Read the model definition and answer for the solid it produces. Units are mm, in the model's axes. A direction names the side the tool comes from. Round coordinates to 2 decimals unless told otherwise and drop trailing zeros. Write each loop counter-clockwise with the first axis right and the second up, starting at its lowest first coordinate (ties: lowest second). Pieces come first, ordered by that corner, then holes. Notation, with made-up numbers: (52.5, 23) - (104.5, 23) arc R22 cw to (104.5, 48) - close; hole circle Ø11 at (62, 43). An arc over 180 degrees is marked (long way). One line per item, written item: value. Start each with the question number.
(1) A cutting plane is placed at A-A, the plane x = -11. Determine the outline of the cut face in (y, z), plus the area to 3 significant figures.
(2) Find the intervals of material crossed by L1, parallel to Y at x = 12.5, z = 9.25; L2, parallel to Z at x = 31, y = -2.4; L3, parallel to X at y = -0.05, z = 0.5, in increasing order.
(3) A cutting plane is placed at C-C, the plane y = -2.3. Determine the outline of the cut face in (x, z).
(4) A cutting plane is placed at B-B, the plane z = 0. Determine the outline of the cut face in (x, y).
(5) For faces 1 (the face through (0, -2, 8)), 2 (the face through (-40.498, -1.986, 0.176)), 3 (the face through (40.498, -1.986, -0.176)), 4 (the face through (0, -2, -8)), determine the directions among +Z, -Z, +X, -X, +Y, -Y from which every point of the face is accessible in a straight line to the end or side of a thin tool.
(6) A flat-ended cylindrical pin translates along its axis: pin 1 Ø0.6 at (x, y) = (-7, -2.5) entering from -Z. Find the tip coordinate at first contact, or state that the pin passes through.
from build123d import *

# Parameters (mm, degrees)
F1_DEPTH = 1
F2_DEPTH = 3


with BuildPart() as f1:
    # F0 (on Front) → F1 (new body)
    with BuildSketch(Plane.XZ):
        with BuildLine():
            Line((-32.5, 8.5), (-32.5, 10.1))
            ThreePointArc((-32.5, 10.1), (-42.6, 0), (-32.5, -10.1))
            Line((-32.5, -10.1), (32.5, -10.1))
            Line((32.5, -10.1), (32.5, -8.5))
            Line((32.5, -8.5), (-32.5, -8.5))
            ThreePointArc((-32.5, -8.5), (-41, 0), (-32.5, 8.5))
        make_face()
        with BuildLine():
            Line((32.5, 10.1), (-32.5, 10.1))
            Line((-32.5, 10.1), (-32.5, 8.5))
            Line((-32.5, 8.5), (32.5, 8.5))
            ThreePointArc((32.5, 8.5), (41, 0), (32.5, -8.5))
            Line((32.5, -8.5), (32.5, -10.1))
            ThreePointArc((32.5, -10.1), (42.6, 0), (32.5, 10.1))
        make_face()
        with BuildLine():
            Line((32.5, 8.5), (-32.5, 8.5))
            Line((-32.5, 8.5), (-32.5, 8))
            Line((-32.5, 8), (32.5, 8))
            ThreePointArc((32.5, 8), (40.5, 0), (32.5, -8))
            Line((32.5, -8), (32.5, -8.5))
            ThreePointArc((32.5, -8.5), (41, 0), (32.5, 8.5))
        make_face()
        with BuildLine():
            Line((-32.5, 8), (-32.5, 8.5))
            ThreePointArc((-32.5, 8.5), (-41, 0), (-32.5, -8.5))
            Line((-32.5, -8.5), (32.5, -8.5))
            Line((32.5, -8.5), (32.5, -8))
            Line((32.5, -8), (-32.5, -8))
            ThreePointArc((-32.5, -8), (-40.5, 0), (-32.5, 8))
        make_face()
    extrude(amount=F1_DEPTH)

    # F0 (on Front) → F2 (join)
    with BuildSketch(Plane.XZ):
        with BuildLine():
            Line((32.5, 8), (-32.5, 8))
            ThreePointArc((-32.5, 8), (-40.5, 0), (-32.5, -8))
            Line((-32.5, -8), (32.5, -8))
            ThreePointArc((32.5, -8), (40.5, 0), (32.5, 8))
        make_face()
    extrude(amount=F2_DEPTH)


solid = f1.part
Here are the results:
1. outline: (-3, -8) - (-1, -8) - (-1, -10.1) - (0, -10.1) - (0, 10.1) - (-1, 10.1) - (-1, 8) - (-3, 8) - close
1. area: 52.2 mm²
2. L1: -1 to 0
2. L2: -8 to 8
2. L3: -42.59 to 42.59
3. outline: (-32.5, -8) - (32.5, -8) arc R8 ccw to (32.5, 8) - (-32.5, 8) arc R8 ccw to start
4. outline: (-42.6, -1) - (-40.5, -1) - (-40.5, -3) - (40.5, -3) - (40.5, -1) - (42.6, -1) - (42.6, 0) - (-42.6, 0) - close
5. face 1: +Z, +X, -X, -Y
5. face 2: -X, -Y
5. face 3: +X, -Y
5. face 4: -Z, +X, -X, -Y
6. pin 1: z = -8
